Geometry check sheet. Reference: the model listing, model coordinates, mm. Round coordinates to 2 decimals unless told otherwise and drop trailing zeros. Loops run counter-clockwise (first coordinate to the right, second up) from the corner with the lowest first, then second, coordinate; pieces in that order, holes last.
```python
from build123d import *

# Parameters (mm, degrees)
BOSS_EXTRUDE1_DEPTH = 3.175
CUT_EXTRUDE1_DEPTH  = 3.175
FILLET1_R           = 6.35
SKETCH3_W           = 63.5
SKETCH3_H           = 3.175
BOSS_EXTRUDE2_DEPTH = 4.7625
CUT_EXTRUDE2_DEPTH  = 386.753713985


with BuildPart() as part:
    # Sketch1 → Boss-Extrude1 (new body)
    with BuildSketch(Plane(origin=(0, 0, 0), x_dir=(1, 0, 0), z_dir=(0, 1, 0))):
        Polygon((0, 301.244), (-17.78, 301.244), (-240.931317375, 0), (-126.631317375, 0), align=None)
    extrude(amount=BOSS_EXTRUDE1_DEPTH)

    # Sketch2 → Cut-Extrude1 (cut)
    with BuildSketch(Plane(origin=(0, 3.175, 0), x_dir=(1, 0, 0), z_dir=(0, 1, 0))):
        Polygon((-143.507037027, 25.4), (-81.84578186, 172.086329549), (-190.506029632, 25.4), align=None)
    extrude(amount=-CUT_EXTRUDE1_DEPTH, mode=Mode.SUBTRACT)

    # Fillet1
    fillet1_edges = [part.edges().sort_by_distance(p)[0] for p in [
        (-143.507037027, 1.5875, -25.4),
        (-190.506029632, 1.5875, -25.4),
        (-81.84578186, 1.5875, -172.086329549),
    ]]
    fillet(fillet1_edges, radius=FILLET1_R)

    # Sketch3 → Boss-Extrude2 (add)
    with BuildSketch(Plane.XY):
        with Locations((-183.781317375, 1.5875)):
            Rectangle(SKETCH3_W, SKETCH3_H)
    extrude(amount=BOSS_EXTRUDE2_DEPTH)

    # Sketch4 → Cut-Extrude2 (cut, through all)
    with BuildSketch(Plane(origin=(0, 3.175, 0), x_dir=(1, 0, 0), z_dir=(0, 1, 0))):
        Polygon((-17.78, 301.244), (-239.661317375, 0), (-240.931317375, 0), align=None)
    extrude(amount=-CUT_EXTRUDE2_DEPTH, mode=Mode.SUBTRACT)


solid = part.part
```
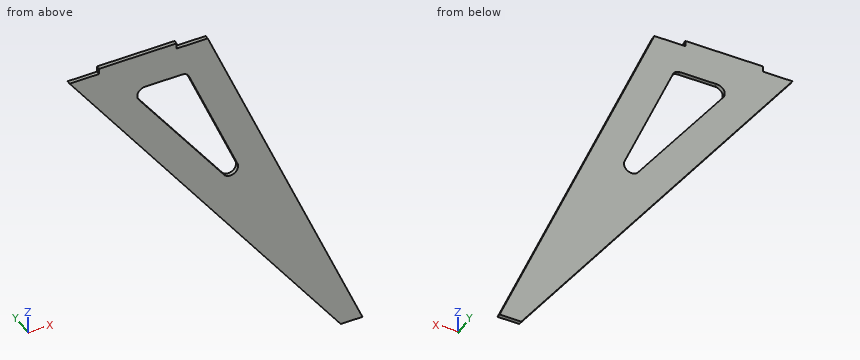
1) Scan lines: line 1 along X through (y, z) = (1.25, -120.5); line 2 along X through (y, z) = (1.3, -46); line 3 along Z through (x, y) = (-168.5, 0.95). Record each from-to range of solid material in increasing order.
Report:
line 1: x = -150.91 to -120.06, -103.53 to -75.98
line 2: x = -205.78 to -175.25, -134.85 to -107.29
line 3: z = -96.61 to -55.11, -25.4 to 4.76
2) Gauge pin test, flat ends, axial feed: pin 1 (1.6 mm diameter, centred on y = 2, z = 3, fed in from +X); pin 2 (1 mm diameter, centred on y = 2.5, z = -89, fed in from +X). Record the tip position at first contact, or that the pin passes through.
Report:
pin 1: stops at x = -152.03
pin 2: stops at x = -89.01
3) Sectioned sample at C-C, the plane x = -164. Record the cut outline in (y, z) (1 decimal).
Report:
outline: (0, -102.7) - (3.2, -102.7) - (3.2, -61.2) - (0, -61.2) - close; (0, -25.4) - (3.2, -25.4) - (3.2, 4.8) - (0, 4.8) - close
4) Sectioned sample at D-D, the plane z = -187. Record the cut outline in (x, y) (3 decimals), then the cut area to 3 significant figures.
Report:
outline: (-101.926, 0) - (-48.024, 0) - (-48.024, 3.175) - (-101.926, 3.175) - close
area: 171 mm2
5) Sectioned sample at A-A, the plane x = -132.5. Record the cut outline in (y, z) (3 decimals), then the cut area to 3 significant figures.
Report:
outline: (0, -145.491) - (3.175, -145.491) - (3.175, -103.705) - (0, -103.705) - close; (0, -51.585) - (3.175, -51.585) - (3.175, 0) - (0, 0) - close
area: 296 mm2
6) Sectioned sample at B-B, the plane y = 2.2. Record the cut outline in (x, z), then the cut area to 3 significant figures.
Report:
outline: (-239.66, 0) - (-17.78, -301.24) - (0, -301.24) - (-126.63, 0) - (-152.03, 0) - (-152.03, 4.76) - (-215.53, 4.76) - (-215.53, 0) - close; hole (-183, -35.53) - (-113.24, -129.7) arc R6.35 ccw to (-102.29, -123.46) - (-141.87, -29.29) arc R6.35 ccw to (-147.73, -25.4) - (-177.9, -25.4) arc R6.35 ccw to start
area: 16,900 mm2
